For this review, take the finished solid that the model builds, in its own axes (mm). Coordinates: 2 decimals unless noted, no trailing zeros. Loops run counter-clockwise (first coordinate to the right, second up) from the corner with the lowest first, then second, coordinate; pieces in that order, holes last. Notation, with made-up numbers: M 26,56 L 40,56 A21 cw 40,79 Z; hole C 86,66 d10. An arc over 180 degrees is marked long. Use one line per item in the form item = value.
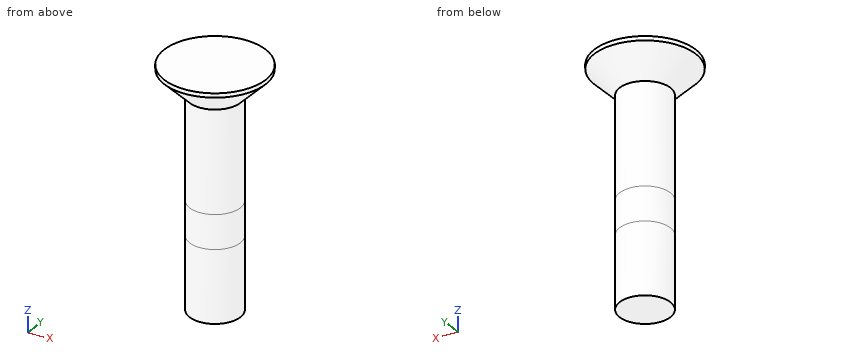
Autodesk Inventor part; units mm, degrees
ref_plane "YZ Plane" through (0, 0, 0) normal (1, 0, 0) x (0, 1, 0)
ref_plane "XZ Plane" through (0, 0, 0) normal (0, 1, 0) x (-1, 0, 0)
ref_plane "XY Plane" through (0, 0, 0) normal (0, 0, 1) x (1, 0, 0)
sketch "スケッチ1" plane through (0, 0, 0) normal (0, 0, 1) x (1, 0, 0)
  circle A0 centre (0, 0) radius 1.5
  dimension "d0" = 3
extrude "押し出し1" add sketch "スケッチ1" along normal blind 6
sketch "スケッチ2" plane through (0, 0, 6) normal (0, 0, 1) x (1, 0, 0)
  circle A0 centre (0, 0) radius 1.5
  circle A1 centre (0, 0) radius 3
  dimension "d3" = 6
extrude "押し出し2" add sketch "スケッチ2" along normal blind 1.75 contours A0 | A1
thread "ねじ1"
chamfer "面取り1" distance 1.5 angle 45 1 edges at (-3, 0, 6)
sketch "スケッチ4" plane through (0, 0, 0) normal (0, 0, -1) x (-1, 0, 0)
  circle A0 centre (0, 0) radius 1.5
extrude "押し出し4" add sketch "スケッチ4" along normal blind 4
sketch "スケッチ5" plane through (0, 0, -4) normal (0, 0, -1) x (-1, 0, 0)
  circle A0 centre (0, 0) radius 1.5
extrude "押し出し5" cut sketch "スケッチ5" against normal blind 2
sketch "スケッチ6" plane through (0, 0, -2) normal (0, 0, -1) x (-1, 0, 0)
  circle A0 centre (0, 0) radius 1.5
extrude "押し出し6" add sketch "スケッチ6" along normal blind 4.25
properties part number "SB　14mm皿ネジ" material "Steel, Mild"
1. Consider section C-C on z = -1.25. Write out the cut boundary in (x, y).
Computed values:
outline = C 0,0 d3
2. Wall thickness on line 1 along X through (y, z) = (-0.95, 5.5); line 2 along Z through (x, y) = (-2.4, -1.75); line 3 along Y through (x, z) = (-0.35, -0.25): over which ranges is each line inside the solid? List them lowest first. Write a range as from..to.
Computed values:
line_1 = -1.16..1.16
line_2 = 7.47..7.75
line_3 = -1.46..1.46
3. For pin 1 Ø3 at (y, z) = (1.5, 2) entering from -X; pin 2 Ø2 at (y, z) = (-1, -3.5) entering from +X; pin 3 Ø1.5 at (y, z) = (2, 4.5) entering from +X, all flat-tipped, find the tip position at first contact; note any pin that passes through.
Computed values:
pin_1 = -1.5
pin_2 = 1.5
pin_3 = 0.83
